Could you check a few things on this drawing? It's one solid part, dimensions in mm from its lowest x, y, z. A direction names the side the tool comes from. Give positions to 0.01 mm unless a question says otherwise; leave off trailing zeros. Order: outer loops, then holes, each group sorted by start corner. A loop starts at its lowest first (then second) coordinate and runs counter-clockwise, first axis right, second up. Notation, with made-up numbers: (-27.75, -33) - (-1.75, -33) arc R23 ccw to (-1.75, 4) - close; hole circle Ø4 at (28, -32.5). An arc over 180 degrees is marked (long way). Put each result on its own line as item: value.
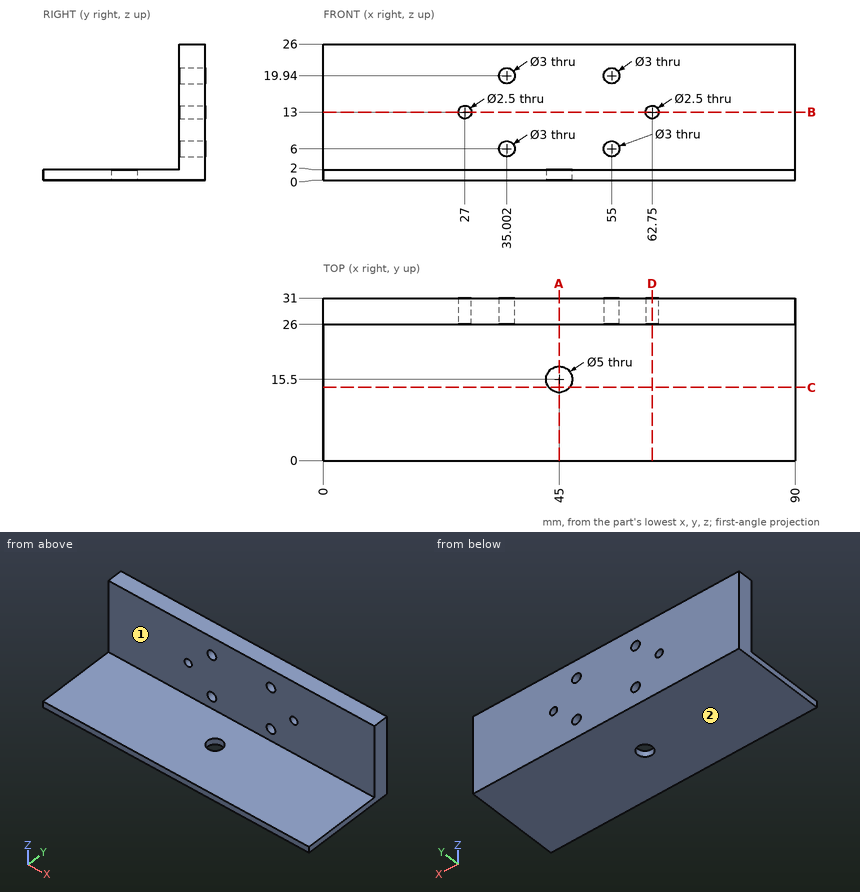
1) Which directions (+Z, -Z, +X, -X, +Y, -Y) give clear straight access to the entire face, cutting with the end or side of a thin tool? Please do the marked faces 1 and 2.
Filled in:
face 1: +Z, +X, -X, -Y
face 2: -Z, +X, -X, +Y, -Y
2) If I drill on line 1 (Y direction, x = 48.5, z = 5); line 2 (Z direction, x = 34.5, y = 16); line 3 (Z direction, x = 62, y = 29), over which ranges is the centre line in solid material (lowest first)? Write a range as [from, to].
Filled in:
line 1: y = [26, 31]
line 2: z = [0, 2]
line 3: z = [0, 12], [14, 26]
3) I'm going to push flat-ended pins straight in: pin 1 (5 mm diameter, centred on x = 30, z = 13.5, fed in from -Y); pin 2 (2.5 mm diameter, centred on x = 55, z = 6, fed in from -Y). Where does each tip first touch, or does it pass through?
Filled in:
pin 1: stops at y = 26
pin 2: passes through
4) Suppose I cut it at D-D, the plane x = 62.75. List the corners of the cut face in (y, z) for me.
Filled in:
outline: (0, 0) - (31, 0) - (31, 11.75) - (26, 11.75) - (26, 2) - (0, 2) - close; (26, 14.25) - (31, 14.25) - (31, 26) - (26, 26) - close
5) Suppose I cut it at C-C, the plane y = 14. List the corners of the cut face in (x, z) for me, and give its area (3 significant figures).
Filled in:
outline: (0, 0) - (43, 0) - (43, 2) - (0, 2) - close; (47, 0) - (90, 0) - (90, 2) - (47, 2) - close
area: 172 mm^2
6) Suppose I cut it at A-A, the plane x = 45. List the corners of the cut face in (y, z) for me.
Filled in:
outline: (0, 0) - (13, 0) - (13, 2) - (0, 2) - close; (18, 0) - (31, 0) - (31, 26) - (26, 26) - (26, 2) - (18, 2) - close
7) Suppose I cut it at B-B, the plane z = 13. List the corners of the cut face in (x, y) for me, and give its area (3 significant figures).
Filled in:
outline: (0, 26) - (25.75, 26) - (25.75, 31) - (0, 31) - close; (28.25, 26) - (61.5, 26) - (61.5, 31) - (28.25, 31) - close; (64, 26) - (90, 26) - (90, 31) - (64, 31) - close
area: 425 mm^2
